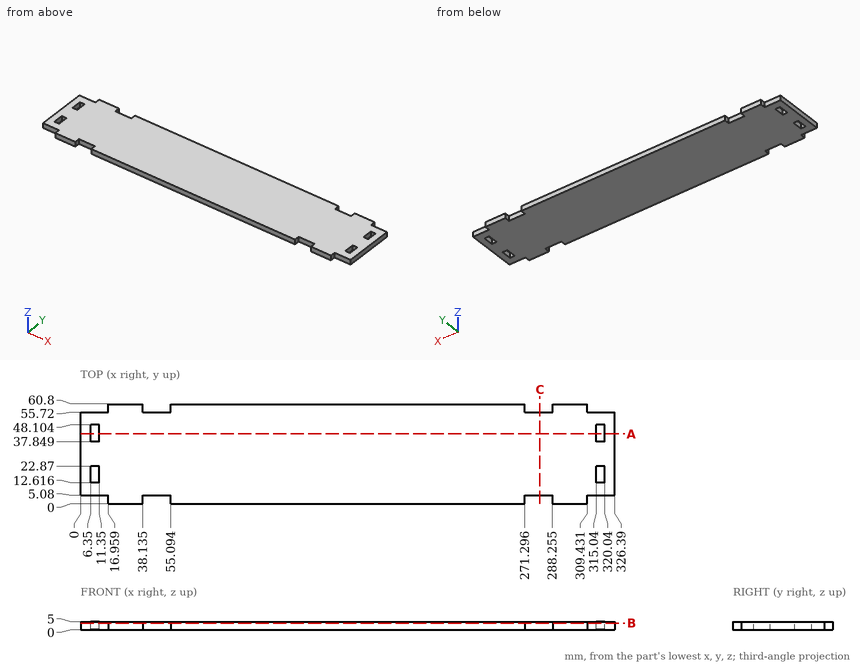
Job drawing, mm, ordinate dimensions from the low corner. One solid piece. Coordinates: 2 decimals unless noted, no trailing zeros. Order: outer loops, then holes, each group sorted by start corner. A loop starts at its lowest first (then second) coordinate and runs counter-clockwise, first axis right, second up. Notation, with made-up numbers: (-25.75, -15) - (2.25, -15) arc R17 ccw to (2.25, -2) - close; hole circle Ø6 at (68.25, 55.5). An arc over 180 degrees is marked (long way). Return JSON: item names as keys, results as strings. Group by question number.
1) Probe line 1 (X direction, y = 5, z = 0.35) (1 decimal); line 2 (X direction, y = 47.5, z = 1.3). List the from-to ranges inside material, lowest first. Write a range as from..to.
2) Saw through at B-B, the plane z = 4.1. Count the separate pieces of the cut face and the enclosed holes in it, plus the area to 4 significant figures.
3) Flat gauge pins, fed straight in: P1, Ø1.5, axis at x = 8.5, z = 3, coming from the -Y side; P2, Ø1.5, axis at x = 44.5, z = 3, coming from the +Y side; P3, Ø1.5, axis at y = 3, z = 3.5, coming from the -X side. Where does each tip first touch, or does it go through?
4) Saw through at A-A, the plane y = 42.5. Write the cut outline in (x, z).
5) Saw through at C-C, the plane x = 280.5. Write the cut outline in (y, z), plus the area to 3 significant figures.
Values found:
{
 "1": {"line 1": "x = 17..38.1, 55.1..271.3, 288.3..309.4", "line 2": "x = 0..6.35, 11.35..315.04, 320.04..326.39"},
 "2": {"separate pieces": "1", "enclosed holes": "4", "area": "18,950 mm²"},
 "3": {"P1": "stops at y = 5.08", "P2": "stops at y = 55.72", "P3": "stops at x = 16.96"},
 "4": {"outline": "(0, 0) - (6.35, 0) - (6.35, 5) - (0, 5) - close; (11.35, 0) - (315.04, 0) - (315.04, 5) - (11.35, 5) - close; (320.04, 0) - (326.39, 0) - (326.39, 5) - (320.04, 5) - close"},
 "5": {"outline": "(5.08, 0) - (55.72, 0) - (55.72, 5) - (5.08, 5) - close", "area": "253 mm²"}
}
